For this review, take the finished solid that the model builds, in its own axes (mm). Face numbers are marked on the shaded views. Round coordinates to 2 decimals unless told otherwise and drop trailing zeros. Loops run counter-clockwise (first coordinate to the right, second up) from the corner with the lowest first, then second, coordinate; pieces in that order, holes last.
1. Consider section D-D on x = -35.75. State the section outline as (y, z) points, then the cut area to 3 significant figures.
2. Consider section B-B on y = -50. State the section outline as (x, z) points.
3. Draft analysis for pull direction Y (two halves, no side actions). For the marked faces 1, 2 and 3, state which applies: released by +Y, released by -Y, zero draft, split by the parting line, or undercut.
4. Clearance check with flat-ended pins moving along their axes: pin 1 Ø1 at (x, z) = (0, 1) entering from -Y; pin 2 Ø5 at (y, z) = (8, 0) entering from -X; pin 3 Ø2 at (x, y) = (0, 0) entering from -Z; pin 4 Ø1.8 at (y, z) = (5, 8.5) entering from +X. State where each tip first meets the part, or that it passes through.
5. To check wall thickness, follow line 1 along Y through (x, z) = (-35.75, -0.3); line 2 along Y through (x, z) = (0, 5); line 3 along X through (y, z) = (8, 1.75). State the ranges of each line that lie inside material, in increasing order.
6. Consider section A-A on x = 0. State the section outline as (y, z) points, then the cut area to 3 significant figures.
from build123d import *

# Parameters (mm, degrees)
SKICA1_W                     = 50
SKICA1_H                     = 50
P_IDAT_VYSUNUT_M1_DEPTH      = 10
ODEBRAT_VYSUNUT_M2_DEPTH     = 57.789083458
P_IDAT_VYSUNUT_M4_DEPTH      = 1
P_IDAT_VYSUNUT_M4_DEPTH_BACK = 2.5
SKICA4_R                     = 2
SKICA4_W                     = 50
SKICA4_H                     = 50
SKICA6_R                     = 1.85
ODEBRAT_VYSUNUT_M3_DEPTH     = 71.416176377
SKICA7_W                     = 50
SKICA7_H                     = 1
ODEBRAT_VYSUNUT_M4_DEPTH     = 92.446366224
SKICA9_W                     = 6.5
SKICA9_H                     = 3.727272727
ODEBRAT_VYSUNUT_M6_DEPTH     = 88.211595424
ZKOSEN_2_SIZE                = 0.5
P_IDAT_START                 = 0.5
SKICA10_W                    = 9.4
SKICA10_H                    = 46.272727273
SKICA10_R                    = 1.85
SKICA10_W_2                  = 9.7
P_IDAT_VYSUNUT_M5_DEPTH      = 0.5
ZKOSEN_3_SIZE                = 1


with BuildPart() as part:
    # Skica1 → Přidat vysunutím1 (new body)
    with BuildSketch(Plane.XY):
        Rectangle(SKICA1_W, SKICA1_H)
    extrude(amount=P_IDAT_VYSUNUT_M1_DEPTH)

    # Skica3 → Odebrat vysunutím2 (cut, through all)
    with BuildSketch(Plane(origin=(0, 25, 0), x_dir=(1, 0, 0), z_dir=(0, 1, 0))):
        Polygon((-15.3, -10), (-15.3, -7.22080893), (-14.133651513, -5.83080893), (-14.133651513, -5.49919107), (-15.3, -4.10919107), (-15.3, -3.430543964), (-14.999456036, -3.13), (-5.000543964, -3.13), (-4.7, -3.430543964), (-4.7, -4.10919107), (-5.866348487, -5.49919107), (-5.866348487, -5.83080893), (-4.7, -7.22080893), (-4.7, -10), align=None)
        Polygon((15.3, -3.430543964), (14.999456036, -3.13), (5.000543964, -3.13), (4.7, -3.430543964), (4.7, -4.10919107), (5.866348487, -5.49919107), (5.866348487, -5.83080893), (4.7, -7.22080893), (4.7, -10), (15.3, -10), (15.3, -7.22080893), (14.133651513, -5.83080893), (14.133651513, -5.49919107), (15.3, -4.10919107), align=None)
    extrude(amount=-ODEBRAT_VYSUNUT_M2_DEPTH, mode=Mode.SUBTRACT)

    # Skica4 → Přidat vysunutím4 (add, two sides: drawn at the far end of the back side and taken through both)
    # profile 1 of 5: a face of its own
    with BuildSketch(Plane(origin=(0, 0, 0), x_dir=(-1, 0, 0), z_dir=(0, 0, -1)).offset(-P_IDAT_VYSUNUT_M4_DEPTH_BACK)):
        Polygon((-30.25, -56), (-8.085, -25), (-25, -25), (-25, -21.272727273), (-41.248489616, -43.997887574), (-41.248489616, -46.002224154), (-41.248489616, -53.002224154), (-38.25, -56), align=None)
        with Locations((-35.75, -50)):
            Circle(SKICA4_R, mode=Mode.SUBTRACT)
    # profile 2 of 5: a face of its own
    with BuildSketch(Plane(origin=(0, 0, 0), x_dir=(-1, 0, 0), z_dir=(0, 0, -1)).offset(-P_IDAT_VYSUNUT_M4_DEPTH_BACK)):
        Rectangle(SKICA4_W, SKICA4_H)
    # profile 3 of 5: a face of its own
    with BuildSketch(Plane(origin=(0, 0, 0), x_dir=(-1, 0, 0), z_dir=(0, 0, -1)).offset(-P_IDAT_VYSUNUT_M4_DEPTH_BACK)):
        Polygon((-25, 25), (-8.085, 25), (-30.25, 56), (-38.25, 56), (-41.248489616, 53.002224154), (-41.248489616, 46.002224154), (-41.248489616, 43.997887574), (-25, 21.272727273), align=None)
        with Locations((-35.75, 50)):
            Circle(SKICA4_R, mode=Mode.SUBTRACT)
    # profile 4 of 5: a face of its own
    with BuildSketch(Plane(origin=(0, 0, 0), x_dir=(-1, 0, 0), z_dir=(0, 0, -1)).offset(-P_IDAT_VYSUNUT_M4_DEPTH_BACK)):
        Polygon((41.248489616, 46.002224154), (41.248489616, 53.002224154), (38.25, 56), (30.25, 56), (8.085, 25), (25, 25), (25, 21.272727273), (41.248489616, 43.997887574), align=None)
        with Locations((35.75, 50)):
            Circle(SKICA4_R, mode=Mode.SUBTRACT)
    # profile 5 of 5: a face of its own
    with BuildSketch(Plane(origin=(0, 0, 0), x_dir=(-1, 0, 0), z_dir=(0, 0, -1)).offset(-P_IDAT_VYSUNUT_M4_DEPTH_BACK)):
        Polygon((41.248489616, -43.997887574), (25, -21.272727273), (25, -25), (8.085, -25), (30.25, -56), (38.25, -56), (41.248489616, -53.002224154), (41.248489616, -46.002224154), align=None)
        with Locations((35.75, -50)):
            Circle(SKICA4_R, mode=Mode.SUBTRACT)
    extrude(amount=P_IDAT_VYSUNUT_M4_DEPTH + P_IDAT_VYSUNUT_M4_DEPTH_BACK)

    # Skica6 → Odebrat vysunutím3 (cut, through all)
    with BuildSketch(Plane.XY.offset(10)):
        Circle(SKICA6_R)
    extrude(amount=-ODEBRAT_VYSUNUT_M3_DEPTH, mode=Mode.SUBTRACT)

    # Skica7 → Odebrat vysunutím4 (cut, through all)
    with BuildSketch(Plane(origin=(0, 25, 0), x_dir=(1, 0, 0), z_dir=(0, 1, 0))):
        with Locations((0, -9.5)):
            Rectangle(SKICA7_W, SKICA7_H)
    extrude(amount=-ODEBRAT_VYSUNUT_M4_DEPTH, mode=Mode.SUBTRACT)

    # Skica9 → Odebrat vysunutím6 (cut, through all)
    with BuildSketch(Plane(origin=(25, 0, 0), x_dir=(0, 0, -1), z_dir=(1, 0, 0))):
        with Locations((-5.75, -23.136363637)):
            Rectangle(SKICA9_W, SKICA9_H)
    extrude(amount=-ODEBRAT_VYSUNUT_M6_DEPTH, mode=Mode.SUBTRACT)

    # Zkosení2
    zkosen_2_edges = [part.edges().sort_by_distance(p)[0] for p in [
        (-33.75, 50, 2.5),
        (37.75, -50, 2.5),
        (-33.75, -50, 2.5),
        (37.75, 50, 2.5),
    ]]
    chamfer(zkosen_2_edges, length=ZKOSEN_2_SIZE)

    # Skica10 → Přidat vysunutím5 (add)
    # profile 1 of 3: a face of its own
    with BuildSketch(Plane.XY.offset(9).offset(P_IDAT_START)):
        with Locations((0, 1.863636363)):
            Rectangle(SKICA10_W, SKICA10_H)
        Circle(SKICA10_R, mode=Mode.SUBTRACT)
    # profile 2 of 3: a face of its own
    with BuildSketch(Plane.XY.offset(9).offset(P_IDAT_START)):
        with Locations((-20.15, 1.863636363)):
            Rectangle(SKICA10_W_2, SKICA10_H)
    # profile 3 of 3: a face of its own
    with BuildSketch(Plane.XY.offset(9).offset(P_IDAT_START)):
        with Locations((20.15, 1.863636363)):
            Rectangle(SKICA10_W_2, SKICA10_H)
    extrude(amount=-P_IDAT_VYSUNUT_M5_DEPTH)

    # Zkosení3
    zkosen_3_edges = [part.edges().sort_by_distance(p)[0] for p in [
        (-1.85, 0, 9.5),
    ]]
    chamfer(zkosen_3_edges, length=ZKOSEN_3_SIZE)


solid = part.part
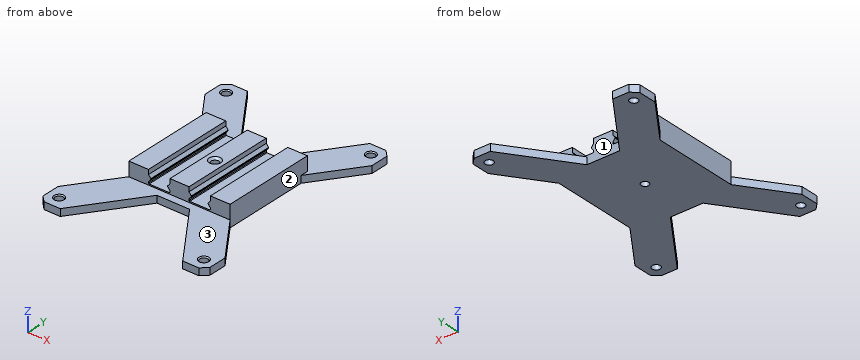
Resolved:
1. outline: (-56, -1) - (-52, -1) - (-52, 2) - (-52.5, 2.5) - (-56, 2.5) - close; (-48, -1) - (-36.31, -1) - (-36.31, 2.5) - (-47.5, 2.5) - (-48, 2) - close; (36.31, -1) - (48, -1) - (48, 2) - (47.5, 2.5) - (36.31, 2.5) - close; (52, -1) - (56, -1) - (56, 2.5) - (52.5, 2.5) - (52, 2) - close
1. area: 109 mm2
2. outline: (-41.25, -1) - (-37.75, -1) - (-37.75, 2) - (-38.25, 2.5) - (-41.25, 2.5) - close; (-33.75, -1) - (-25.96, -1) - (-25.96, 2.5) - (-33.25, 2.5) - (-33.75, 2) - close; (25.96, -1) - (33.75, -1) - (33.75, 2) - (33.25, 2.5) - (25.96, 2.5) - close; (37.75, -1) - (41.25, -1) - (41.25, 2.5) - (38.25, 2.5) - (37.75, 2) - close
3. face 1: released by +Y
3. face 2: undercut
3. face 3: zero draft
4. pin 1: stops at y = -25
4. pin 2: stops at x = -25
4. pin 3: passes through
4. pin 4: stops at x = 25
5. line 1: y = -56 to -52, -48 to -36.31, 36.31 to 48, 52 to 56
5. line 2: y = -21.27 to -1.85, 1.85 to 25
5. line 3: x = -25 to 25
6. outline: (-25, -1) - (-1.85, -1) - (-1.85, 8.5) - (-2.85, 9.5) - (-21.27, 9.5) - (-21.27, 2.5) - (-25, 2.5) - close; (1.85, -1) - (25, -1) - (25, 9.5) - (2.85, 9.5) - (1.85, 8.5) - close
6. area: 459 mm2
